```python
from build123d import *

# Parameters (mm, degrees)
SKETCH_1_R      = 1.5
EXTRUDE_1_DEPTH = 5.6


with BuildPart() as part:
    # 草图1 → 凸台-拉伸1 (new body)
    with BuildSketch(Plane.XY):
        with BuildLine():
            ThreePointArc((-17.321428571, -2.493614294), (-11.45887756, -13.226644513), (0, -17.5))
            ThreePointArc((0, -17.5), (11.45887756, -13.226644513), (17.321428571, -2.493614294))
            ThreePointArc((17.321428571, -2.493614294), (15, 0), (17.321428571, 2.493614294))
            ThreePointArc((17.321428571, 2.493614294), (0, 17.5), (-17.321428571, 2.493614294))
            ThreePointArc((-17.321428571, 2.493614294), (-15.670187363, 1.70346286), (-15, 0))
            ThreePointArc((-15, 0), (-15.670187363, -1.70346286), (-17.321428571, -2.493614294))
        make_face()
        with Locations((-11.691342951, -6.75)):
            Circle(SKETCH_1_R, mode=Mode.SUBTRACT)
        with BuildLine():
            ThreePointArc((0, -15), (-1.5, -13.5), (0, -12))
            ThreePointArc((0, -12), (1.060660172, -12.439339828), (1.5, -13.5))
            ThreePointArc((1.5, -13.5), (1.060660172, -14.560660172), (0, -15))
        make_face(mode=Mode.SUBTRACT)
        with Locations((11.691342951, -6.75)):
            Circle(SKETCH_1_R, mode=Mode.SUBTRACT)
        with Locations((-11.691342951, 6.75)):
            Circle(SKETCH_1_R, mode=Mode.SUBTRACT)
        with BuildLine():
            ThreePointArc((9, 0), (6.363961031, -6.363961031), (0, -9))
            ThreePointArc((0, -9), (-6.363961031, 6.363961031), (9, 0))
        make_face(mode=Mode.SUBTRACT)
        with Locations((11.691342951, 6.75)):
            Circle(SKETCH_1_R, mode=Mode.SUBTRACT)
        with Locations((0, 13.5)):
            Circle(SKETCH_1_R, mode=Mode.SUBTRACT)
    extrude(amount=EXTRUDE_1_DEPTH)


solid = part.part
```
Work out the finished part from the listing and answer in its coordinate system (mm). Give positions to 0.01 mm unless a question says otherwise; leave off trailing zeros. Loops run counter-clockwise (first coordinate to the right, second up) from the corner with the lowest first, then second, coordinate; pieces in that order, holes last. Notation, with made-up numbers: (67.5, 34) - (71.5, 34) arc R7 cw to (71.5, 47) - close; hole circle Ø1 at (75.25, -25). An arc over 180 degrees is marked (long way). Use CSV: the item, a comma, the result in double quotes. Start each with the question number.
(1) Determine the mould class of faces 1 (the face through (0.35, 17.497, 2.761)), 2 (the face through (13.08, -7.32, 2.76)), 3 (the face through (7, -8, 5.6)) for opening direction Y: released by +Y, released by -Y, zero draft, split by the parting line, or undercut.
(2) Find section B-B, the plane y = 2. Determine the outline of the cut face in (x, z), plus the area to 3 significant figures.
(3) This flat-tipped pin is pushed along its axis until it touches: pin 1 (1 mm diameter, centred on x = -3, z = 2.5, fed in from +Y). Where does it stop, or does it pass through?
(4) Find section D-D, the plane y = 6.75. Determine the outline of the cut face in (x, z), plus the area to 3 significant figures.
(5) Find the intervals of material crossed by L1, parallel to X at y = 6, z = 3.55; L2, parallel to X at y = -7, z = 2.1; L3, parallel to X at y = -4, z = 1.95, in increasing order.
(6) Find section A-A, the plane z = 3.75. Determine the outline of the cut face in (x, y), plus the area to 3 significant figures.
(7) Find section C-C, the plane x = -7. Determine the outline of the cut face in (y, z).
Results found:
1,face 1,"released by +Y"
1,face 2,"undercut"
1,face 3,"zero draft"
2,outline,"(-16, 0) - (-8.77, 0) - (-8.77, 5.6) - (-16, 5.6) - close; (8.77, 0) - (16, 0) - (16, 5.6) - (8.77, 5.6) - close"
2,area,"80.9 mm^2"
3,pin 1,"y = 17.32"
4,outline,"(-16.15, 0) - (-13.19, 0) - (-13.19, 5.6) - (-16.15, 5.6) - close; (-10.19, 0) - (-5.95, 0) - (-5.95, 5.6) - (-10.19, 5.6) - close; (5.95, 0) - (10.19, 0) - (10.19, 5.6) - (5.95, 5.6) - close; (13.19, 0) - (16.15, 0) - (16.15, 5.6) - (13.19, 5.6) - close"
4,area,"80.6 mm^2"
5,L1,"-16.44 to -12.99, -10.39 to -6.71, 6.71 to 10.39, 12.99 to 16.44"
5,L2,"-16.04 to -13.17, -10.21 to -5.66, 5.66 to 10.21, 13.17 to 16.04"
5,L3,"-17.04 to -8.06, 8.06 to 17.04"
6,outline,"(-17.32, -2.49) arc R17.5 ccw to (17.32, -2.49) arc R2.5 cw to (17.32, 2.49) arc R17.5 ccw to (-17.32, 2.49) arc R2.5 cw to start; hole circle Ø3 at (-11.69, -6.75); hole circle Ø3 at (-11.69, 6.75); hole circle Ø18 at (0, 0); hole circle Ø3 at (0, -13.5); hole circle Ø3 at (0, 13.5); hole circle Ø3 at (11.69, -6.75); hole circle Ø3 at (11.69, 6.75)"
6,area,"646 mm^2"
7,outline,"(-16.04, 0) - (-5.66, 0) - (-5.66, 5.6) - (-16.04, 5.6) - close; (5.66, 0) - (16.04, 0) - (16.04, 5.6) - (5.66, 5.6) - close"
